from build123d import *

# Parameters (mm, degrees)
F1_DEPTH = 6
F3_DEPTH = 7.001
F4_R     = 4.75
F5_DEPTH = 25


with BuildPart() as f1:
    # F0 (on Front) → F1 (new body, symmetric)
    with BuildSketch(Plane.XZ):
        Polygon((7, 19), (0, 19), (0, 0), (19, 0), (19, 7), (7, 7), align=None)
    extrude(amount=F1_DEPTH, both=True)

    # F2 (on face) → F3 (cut, through all)
    with BuildSketch(Plane.XY.offset(7)):
        with BuildLine():
            ThreePointArc((19, -3.68273), (20.290251, -2.038688), (20.75, 0))
            ThreePointArc((20.75, 0), (20.290251, 2.038688), (19, 3.68273))
            Line((19, 3.68273), (19, -3.68273))
        make_face()
        with BuildLine():
            Line((19, -3.68273), (19, 3.68273))
            ThreePointArc((19, 3.68273), (11.25, 0), (19, -3.68273))
        make_face()
    extrude(amount=-F3_DEPTH, mode=Mode.SUBTRACT)

    # F4 (on face) → F5 (cut)
    with BuildSketch(Plane.YZ.offset(7)):
        with Locations((0, 16)):
            Circle(F4_R)
    extrude(amount=-F5_DEPTH, mode=Mode.SUBTRACT)


solid = f1.part
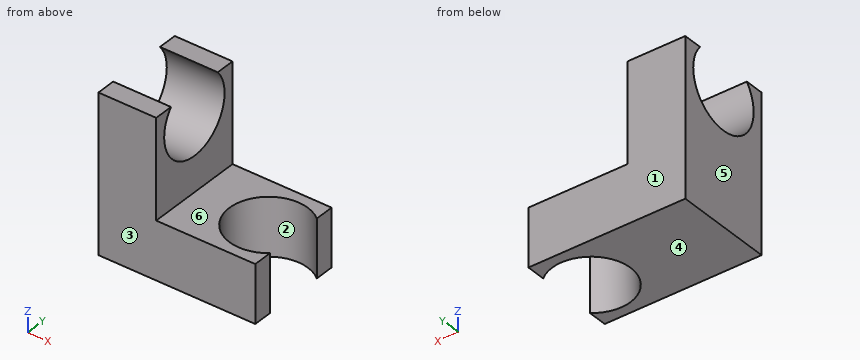
Work out the finished part from the listing and answer in its coordinate system (mm). Face numbers are marked on the shaded views. A direction names the side the tool comes from. Round coordinates to 2 decimals unless told otherwise and drop trailing zeros. Write each loop counter-clockwise with the first axis right and the second up, starting at its lowest first coordinate (ties: lowest second). Pieces come first, ordered by that corner, then holes. Notation, with made-up numbers: (9.25, 29.5) -> (52.25, 29.5) arc R26 ccw to (52.25, 54.5) -> close; hole circle Ø2 at (-28.5, 22). An arc over 180 degrees is marked (long way). Answer as CSV lines item,"result". Start each with the question number.
(1) The mould has two halves that part along Y. Classify the marked faces 1, 2, 3 and 4: +Y half, -Y half, draft (parallel to the pull), parting line (faces both ways), or undercut.
(2) The part is cut by section B-B, the plane z = 16. Give the vertices of the cut face in (x, y).
(3) A tool of negligible diameter and unlimited length cuts with its end or side. For the marked faces 5 and 6, from which of +Z, -Z, +X, -X, +Y, -Y can it reach the whole face along a straight path? Write none if from no direction.
(4) The part is cut by section D-D, the plane z = 2.5. Give the vertices of the cut face in (x, y).
(5) The part is cut by section C-C, the plane y = -5. Give the vertices of the cut face in (x, z).
(6) The part is cut by section A-A, the plane x = 16. Give the vertices of the cut face in (y, z).
(7) Each of these flat-tipped pins is pushed along its axis until it touches: pin 1 (4 mm diameter, centred on x = 5, y = 0, fed in from +Z); pin 2 (3.5 mm diameter, centred on y = -0.5, z = 13.5, fed in from +X) (1 decimal). Where does it stop, or does it pass through?
(8) Find the intervals of material crossed by probe 1 along Y at (x, z) = (16, 4); probe 2 along Y at (x, z) = (3.25, 13); probe 3 along Z at (x, y) = (4, 0), in increasing order.
Output values:
1,face 1,"+Y half"
1,face 2,"undercut"
1,face 3,"-Y half"
1,face 4,"draft"
2,outline,"(0, -6) -> (7, -6) -> (7, -4.75) -> (0, -4.75) -> close; (0, 4.75) -> (7, 4.75) -> (7, 6) -> (0, 6) -> close"
3,face 5,"+Z, -Z, -X, +Y, -Y"
3,face 6,"+Z, +X, +Y, -Y"
4,outline,"(0, -6) -> (19, -6) -> (19, -3.68) arc R4.75 cw (long way) to (19, 3.68) -> (19, 6) -> (0, 6) -> close"
5,outline,"(0, 0) -> (19, 0) -> (19, 7) -> (7, 7) -> (7, 19) -> (0, 19) -> close"
6,outline,"(-6, 0) -> (-4.75, 0) -> (-4.75, 7) -> (-6, 7) -> close; (4.75, 0) -> (6, 0) -> (6, 7) -> (4.75, 7) -> close"
7,pin 1,"stops at z = 11.69"
7,pin 2,"passes through"
8,probe 1,"y = -6 to -4.75, 4.75 to 6"
8,probe 2,"y = -6 to -3.68, 3.68 to 6"
8,probe 3,"z = 0 to 11.25"
